from build123d import *

# Parameters (mm, degrees)
BOSS_EXTRUDE1_OUTLINE_R = 35
BOSS_EXTRUDE1_DEPTH     = 2.5
THICKEN1_T2             = 2
SKETCH7_R               = 37
SKETCH7_R_2             = 33.5
BOSS_EXTRUDE2_DEPTH     = 1


# Read off the part's stored shape, not the designer's step: Boss-Extrude1
with BuildPart() as part:
    # Boss-Extrude1 outline → Boss-Extrude1 (new body)
    with BuildSketch(Plane.XY):
        Circle(BOSS_EXTRUDE1_OUTLINE_R)
        Polygon((-3.181980515, -5.303300859), (-19.692923856, -24.147696578), (-24.147696578, -19.692923856), (-5.303300859, -3.181980515), align=None, mode=Mode.SUBTRACT)
        Polygon((1.5, -6), (3.15, -31), (-3.15, -31), (-1.5, -6), align=None, mode=Mode.SUBTRACT)
        Polygon((5.303300859, -3.181980515), (24.147696578, -19.692923856), (19.692923856, -24.147696578), (3.181980515, -5.303300859), align=None, mode=Mode.SUBTRACT)
        Polygon((-6, -1.5), (-31, -3.15), (-31, 3.15), (-6, 1.5), align=None, mode=Mode.SUBTRACT)
        Polygon((-5.303300859, 3.181980515), (-24.147696578, 19.692923856), (-19.692923856, 24.147696578), (-3.181980515, 5.303300859), align=None, mode=Mode.SUBTRACT)
        Polygon((3.181980515, 5.303300859), (19.692923856, 24.147696578), (24.147696578, 19.692923856), (5.303300859, 3.181980515), align=None, mode=Mode.SUBTRACT)
        Polygon((6, 1.5), (31, 3.15), (31, -3.15), (6, -1.5), align=None, mode=Mode.SUBTRACT)
        Polygon((1.5, 6), (-1.5, 6), (-3.15, 31), (3.15, 31), align=None, mode=Mode.SUBTRACT)
    extrude(amount=BOSS_EXTRUDE1_DEPTH)

    # Surface-Loft3: a surface lofted through 2 sketches
    with BuildLine(Plane.XY.offset(2.5), mode=Mode.PRIVATE) as surface_loft3_1_s0:
        CenterArc((0, 0), 35, 0, 360)
    with BuildLine(Plane.XY.offset(27.5), mode=Mode.PRIVATE) as surface_loft3_1_s1:
        CenterArc((0, 0), 25, 0, 360)
    surface_loft3_1 = Shell.make_loft([surface_loft3_1_s0.wire(), surface_loft3_1_s1.wire()])
    add(Solid.thicken(surface_loft3_1, -THICKEN1_T2))

    # Sketch7 → Boss-Extrude2 (add)
    with BuildSketch(Plane(origin=(0, 0, 2.5), x_dir=(-1, 0, 0), z_dir=(0, 0, -1))):
        Circle(SKETCH7_R)
        Circle(SKETCH7_R_2, mode=Mode.SUBTRACT)
    extrude(amount=BOSS_EXTRUDE2_DEPTH)


solid = part.part
Check sheet for the modelled part. Datum: model origin and axes. Units: mm. A direction names the side the tool comes from. Give positions to 0.01 mm unless a question says otherwise; leave off trailing zeros. Loops run counter-clockwise (first coordinate to the right, second up) from the corner with the lowest first, then second, coordinate; pieces in that order, holes last. Notation, with made-up numbers: M -21.5,49.25 L 5.5,49.25 A17 cw 5.5,64.25 Z; hole C 18,68 d10. An arc over 180 degrees is marked long. Answer as a JSON object with one key per item and string values. Group by question number.
Q1. Go/stop test with flat-tipped pins: P1, Ø2, axis at x = 0, z = 2, coming from the +Y side; P2, Ø2, axis at y = -1.5, z = 1, coming from the +X side; P3, Ø1, axis at x = 5.5, z = 8, coming from the +Y side. Record where each tip stops, or that it passes through.
Q2. Release check for a two-part mould opening along Y. For faces 1 (the flat face through (-31, 0, 1)), 2 (the flat face through (-14, -33, 2.5)) record: released by +Y, released by -Y, zero draft, split by the parting line, or undercut.
Q3. Cross-section at A-A on x = 0. Record the cut outline in (y, z), then the cut area to 3 significant figures.
Q4. Access from +Z, -Z, +X, -X, +Y, -Y to the whole of each face (thin tool, end or side, straight path). Record for faces 3 (the flat face through (14.59, -11.32, 1.23)), 4 (the flat face through (0, 0, 2.5)), 5 (the flat face through (-4.257, -4.228, 1.232)).
Q5. Cross-section at D-D on z = 18.25. Record the cut outline in (x, y).
Q6. Material ranges on line 1 along Z through (x, y) = (30, 18.5); line 2 along Y through (x, z) = (-17, 3.25); line 3 along X through (y, z) = (-16, 24), recorded low to high. Write a range as [from, to].
Q7. Cross-section at B-B on y = 16.5. Give the number of separate pieces and of enclosed holes in the cut face, then the cut area to 3 significant figures.
Evaluation:
{
 "1": {"P1": "stops at y = 37", "P2": "stops at x = 36.99", "P3": "stops at y = 32.55"},
 "2": {"face 1": "undercut", "face 2": "zero draft"},
 "3": {"outline": "M -37,1.5 L -35,1.5 L -35,0 L -31,0 L -31,2.5 L -32.85,2.5 L -23.14,26.76 L -25,27.5 L -35,2.5 L -37,2.5 Z; M -6,0 L 6,0 L 6,2.5 L -6,2.5 Z; M 23.14,26.76 L 32.85,2.5 L 31,2.5 L 31,0 L 35,0 L 35,1.5 L 37,1.5 L 37,2.5 L 35,2.5 L 25,27.5 Z", "area": "160 mm2"},
 "4": {"face 3": "-Z", "face 4": "none", "face 5": "+Z, -Z"},
 "5": {"outline": "C 0,0 d57.4; hole C 0,0 d53.09"},
 "6": {"line 1": "z = [1.5, 2.5]", "line 2": "y = [-30.25, -27.75], [27.75, 30.25]", "line 3": "x = [-21, -18.22], [18.22, 21]"},
 "7": {"separate pieces": "4", "enclosed holes": "0", "area": "241 mm2"}
}
